Here's the drawing with two shaded views (mm, measured from the low corner). I have some questions. Coordinates: 2 decimals unless noted, no trailing zeros. Loops run counter-clockwise (first coordinate to the right, second up) from the corner with the lowest first, then second, coordinate; pieces in that order, holes last. Notation, with made-up numbers: (-20.75, 10) -> (-14.75, 10) arc R29 ccw to (-14.75, 48) -> close; hole circle Ø3 at (80, 5.25). An arc over 180 degrees is marked (long way). Answer as a JSON object with one key per item and string values. Group by question number.
Q1. I want a section at B-B on z = 66. Write out the boundary of the cut face in (x, y).
Q2. I need wall thicknesses on line 1 (Z direction, x = 5.5, y = 1.9); line 2 (X direction, y = 0.4, z = 50.5); line 3 (Z direction, x = 84, y = 1.6). Which ranges of each line are inside material? Lowest first, please.
Q3. I want a section at D-D on y = 2. Count the separate pieces of the cut face and the enclosed holes in it, then the cut area to 3 significant figures.
Q4. I'm going to push flat-ended pins straight in: pin 1 (1.5 mm diameter, centred on y = 1.5, z = 74, fed in from +X); pin 2 (0.9 mm diameter, centred on x = 38.5, y = 2, fed in from +Z). Where does each tip first touch, or does it pass through?
Q5. I want a section at C-C on z = 36.5. Write out the boundary of the cut face in (x, y), then the cut area to 3 significant figures.
Q6. I want a section at A-A on x = 5.5. Write out the boundary of the cut face in (y, z).
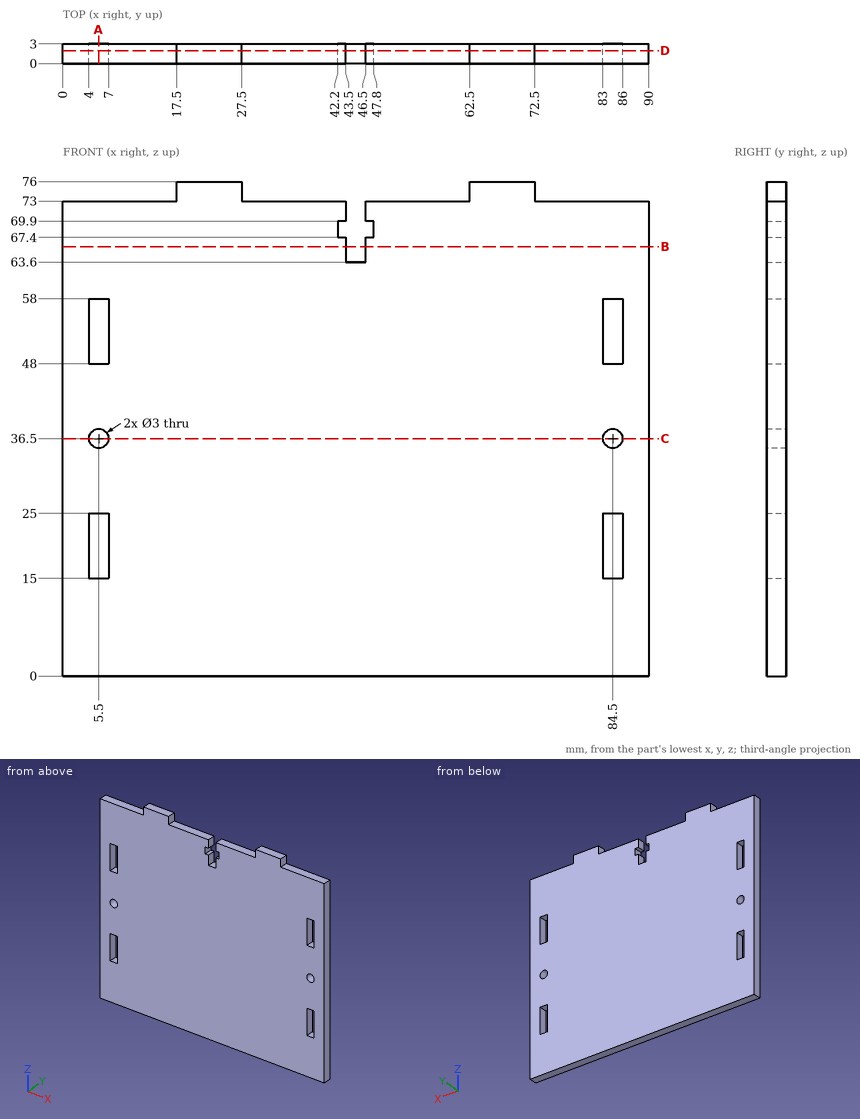
Result set:
{
 "1": {"outline": "(0, 0) -> (43.5, 0) -> (43.5, 3) -> (0, 3) -> close; (46.5, 0) -> (90, 0) -> (90, 3) -> (46.5, 3) -> close"},
 "2": {"line 1": "z = 0 to 15, 25 to 35, 38 to 48, 58 to 73", "line 2": "x = 0 to 4, 7 to 83, 86 to 90", "line 3": "z = 0 to 15, 25 to 35.09, 37.91 to 48, 58 to 73"},
 "3": {"separate pieces": "1", "enclosed holes": "6", "area": "6,460 mm²"},
 "4": {"pin 1": "stops at x = 72.5", "pin 2": "stops at z = 73"},
 "5": {"outline": "(0, 0) -> (4, 0) -> (4, 3) -> (0, 3) -> close; (7, 0) -> (83, 0) -> (83, 3) -> (7, 3) -> close; (86, 0) -> (90, 0) -> (90, 3) -> (86, 3) -> close", "area": "252 mm²"},
 "6": {"outline": "(0, 0) -> (3, 0) -> (3, 15) -> (0, 15) -> close; (0, 25) -> (3, 25) -> (3, 35) -> (0, 35) -> close; (0, 38) -> (3, 38) -> (3, 48) -> (0, 48) -> close; (0, 58) -> (3, 58) -> (3, 73) -> (0, 73) -> close"}
}
